Work out the finished part from the listing and answer in its coordinate system (mm). A direction names the side the tool comes from. Give positions to 0.01 mm unless a question says otherwise; leave off trailing zeros. Loops run counter-clockwise (first coordinate to the right, second up) from the corner with the lowest first, then second, coordinate; pieces in that order, holes last.
```python
from build123d import *

# Parameters (mm, degrees)
F0_W      = 10
F0_H      = 35
F1_DEPTH  = 1
F2_W      = 6
F2_H      = 10
F3_DEPTH  = 3.5
F4_R      = 1.5
F5_DEPTH  = 1
F6_W      = 8.476907853
F6_H      = 3.0214712024
F7_DEPTH  = 2
F8_W      = 0.392
F8_H      = 7
F9_DEPTH  = 0.3
F10_R     = 1.5
F11_DEPTH = 3.301
F12_R     = 0.99999
F13_W     = 6
F13_H     = 0.4
F14_DEPTH = 1.3


# Not quite as in the source:
# - a fillet or chamfer is up to 0.001 mm smaller than in the source, because OpenCascade refuses the exact size


with BuildPart() as f1:
    # F0 (on Top) → F1 (new body)
    with BuildSketch(Plane.XY):
        with Locations((-11.4876428805, 10.5133079179)):
            Rectangle(F0_W, F0_H)
    extrude(amount=F1_DEPTH)

    # F2 (on face) → F3 (join)
    with BuildSketch(Plane.XY.offset(1)):
        with Locations((-11.4876428805, -1.9866920821)):
            Rectangle(F2_W, F2_H)
    extrude(amount=F3_DEPTH)

    # F4 (on face) → F5 (join)
    with BuildSketch(Plane.XY.offset(4.5)):
        with Locations((-11.4072084332, 0)):
            Circle(F4_R)
        with Locations((-11.4072084332, -3.8623050655)):
            Circle(F4_R)
    extrude(amount=F5_DEPTH)

    # F6 (on face) → F7 (join)
    with BuildSketch(Plane(origin=(0, 0, 0), x_dir=(1, 0, 0), z_dir=(0, 0, -1))):
        with Locations((-11.5416448098, -25.7204081863)):
            Rectangle(F6_W, F6_H)
    extrude(amount=F7_DEPTH)

    # F8 (on face) → F9 (join)
    with BuildSketch(Plane(origin=(0, 0, -2), x_dir=(1, 0, 0), z_dir=(0, 0, -1))):
        with Locations((-14.1843358078, -29.2204081863)):
            Rectangle(F8_W, F8_H)
        with Locations((-11.8782826397, -29.261767303)):
            Rectangle(F8_W, F8_H)
        with Locations((-9.3856059038, -29.2204081863)):
            Rectangle(F8_W, F8_H)
    extrude(amount=F9_DEPTH)

    # F10 (on face) → F11 (cut, through all)
    with BuildSketch(Plane.XY.offset(1)):
        with Locations((-11.4876428805, 10.0133079179)):
            Circle(F10_R)
    extrude(amount=-F11_DEPTH, mode=Mode.SUBTRACT)

    # F12 (radius 1 in the source; OpenCascade refuses exactly that, so slightly less here)
    f12_edges = [f1.edges().sort_by_distance(p)[0] for p in [
        (-12.907208, -3.862305, 5.5),
        (-12.907208, 0, 5.5),
    ]]
    fillet(f12_edges, radius=F12_R)

    # F13 (on face) → F14 (join)
    with BuildSketch(Plane.XY.offset(4.5)):
        with Locations((-11.4876428805, -1.9866920821)):
            Rectangle(F13_W, F13_H)
    extrude(amount=F14_DEPTH)


solid = f1.part
```
Q1. Which of the six approach directions +Z, -Z, +X, -X, +Y, -Y give full straight-line access (tool end or side, diameter ignored) to faces 1 (the face through (-12, 24.21, -1)), 2 (the face through (-15.78, 26, -1)), 3 (the face through (-11.4, 0, 5.5))?
Q2. Section B-B on x = -7.75 is taken. Give the vertices of the cut face in (y, z).
Q3. Given pin 1 (4 mm diameter, centred on y = 24, z = 1.5, fed in from +X); pin 2 (1.4 mm diameter, centred on x = -11.5, y = -5.5, fed in from +Z); pin 3 (5 mm diameter, centred on x = -13, y = 12, fed in from -Z); pin 4 (1.8 mm diameter, centred on x = -10.5, z = 2.5, fed in from +Y), each flat-ended and moving along its own axis, determine where each tip first touches the part or whether it passes through.
Q4. Consider line 1 along Y through (x, z) = (-11.5, 0.75); line 2 along Z through (x, y) = (-15.25, 9); line 3 along X through (y, z) = (25.5, -0.5). Determine where each line is inside the solid, lowest interval first.
Q5. Section D-D on y = 6 is taken. Give the vertices of the cut face in (x, z), plus the area to 3 significant figures.
Q6. Section A-A on y = 10.5 is taken. Give the vertices of the cut face in (x, z).
Q7. Determine the mould class of faces 4 (the face through (-12, 25, -2)), 5 (the face through (-10.681, 11.278, 0.507)), 6 (the face through (-12, 3.013, 3)), 7 (the face through (-12, -6.987, 2)) for opening direction Y: +Y half, -Y half, draft (parallel to the pull), parting line (faces both ways), or undercut.
Q8. Section C-C on z = 1.75 is taken. Give the vertices of the cut face in (x, y).
Check result:
1. face 1: -Z, +X, -X, -Y
1. face 2: -Z, -X, +Y, -Y
1. face 3: +Z, +X, -X, +Y
2. outline: (-6.99, 0) - (24.21, 0) - (24.21, -2) - (27.23, -2) - (27.23, 0) - (28.01, 0) - (28.01, 1) - (-6.99, 1) - close
3. pin 1: stops at x = -6.49
3. pin 2: stops at z = 5.4
3. pin 3: stops at z = 0
3. pin 4: stops at y = 3.01
4. line 1: y = -6.99 to 8.51, 11.51 to 28.01
4. line 2: z = 0 to 1
4. line 3: x = -15.78 to -7.3
5. outline: (-16.49, 0) - (-6.49, 0) - (-6.49, 1) - (-16.49, 1) - close
5. area: 10.0 mm2
6. outline: (-16.49, 0) - (-12.91, 0) - (-12.91, 1) - (-16.49, 1) - close; (-10.07, 0) - (-6.49, 0) - (-6.49, 1) - (-10.07, 1) - close
7. face 4: draft
7. face 5: undercut
7. face 6: +Y half
7. face 7: -Y half
8. outline: (-14.49, -6.99) - (-8.49, -6.99) - (-8.49, 3.01) - (-14.49, 3.01) - close
